Read the model definition and answer for the solid it produces. Units are mm, in the model's axes. Round coordinates to 2 decimals unless told otherwise and drop trailing zeros. One line per item, written item: value. Start each with the question number.
1. Consider line 1 (X direction, y = 77.5, z = 1.5); line 2 (Y direction, x = -30, z = 4.25); line 3 (Y direction, x = -64.5, z = 1.25). Determine where each line is inside the solid, lowest interval first.
2. The mould has two halves that part along Y. Classify faces 1 (the face through (-27, 109, 0.2)), 2 (the face through (-27, 100, 0.2)), 3 (the face through (3.05, -40.42, 4.45)), 4 (the face through (2.93, 118.42, 4.45)): released by +Y, released by -Y, zero draft, split by the parting line, or undercut.
3. Flat-ended cylindrical pins translate along their axes: pin 1 Ø3 at (y, z) = (-12, 5) entering from +X; pin 2 Ø1.1 at (x, z) = (-19.5, 4.5) entering from -Y; pin 3 Ø0.6 at (y, z) = (-42, 4.5) entering from -X. Find the tip coordinate at first contact, or state that the pin passes through.
from build123d import *

# Parameters (mm, degrees)
EXTRUDE_2_DEPTH     = 7.99
FILLET_4_R          = 1
EXTRUDE_4_DEPTH     = 0.7
SKETCH_13_R         = 0.94846709
CUT_EXTRUDE_2_DEPTH = 1
CUT_EXTRUDE_3_DEPTH = 1.5
CUT_EXTRUDE_4_DEPTH = 1.5
CUT_EXTRUDE_6_DEPTH = 0.2


with BuildPart() as part:
    # 草图1 → 凸台-拉伸2 (new body)
    with BuildSketch(Plane.XY):
        with BuildLine():
            Line((-62.348303156, 120.705678339), (-2.668303156, 120.705678339))
            ThreePointArc((-2.668303156, 120.705678339), (2.988551094, 118.362532589), (5.331696844, 112.705678339))
            Line((5.331696844, 112.705678339), (5.331696844, -34.824321661))
            ThreePointArc((5.331696844, -34.824321661), (2.988551094, -40.48117591), (-2.668303156, -42.824321661))
            Line((-2.668303156, -42.824321661), (-62.348303156, -42.824321661))
            ThreePointArc((-62.348303156, -42.824321661), (-68.005157405, -40.48117591), (-70.348303156, -34.824321661))
            Line((-70.348303156, -34.824321661), (-70.348303156, 112.705678339))
            ThreePointArc((-70.348303156, 112.705678339), (-68.005157405, 118.362532589), (-62.348303156, 120.705678339))
        make_face()
    extrude(amount=EXTRUDE_2_DEPTH)

    # 圆角4
    fillet_4_edges = [part.edges().sort_by_distance(p)[0] for p in [
        (5.331696844, 38.940678339, 0),
        (2.988551094, -40.48117591, 0),
        (-32.508303156, -42.824321661, 0),
        (-68.005157405, -40.48117591, 0),
        (-70.348303156, 38.940678339, 0),
        (-68.005157405, 118.362532589, 0),
        (-32.508303156, 120.705678339, 0),
        (2.988551094, 118.362532589, 0),
    ]]
    fillet(fillet_4_edges, radius=FILLET_4_R)

    # 草图7 → 凸台-拉伸4 (add)
    with BuildSketch(Plane(origin=(5.331696844, -15.049624304, 0), x_dir=(0, 0, -1), z_dir=(1, 0, 0))):
        with BuildLine():
            Line((-4.598017409, 67.245409355), (-4.480245782, 67.245409355))
            ThreePointArc((-4.480245782, 67.245409355), (-3.41958561, 66.806069527), (-2.980245782, 65.745409355))
            Line((-2.980245782, 65.745409355), (-2.980245782, 58.745409355))
            ThreePointArc((-2.980245782, 58.745409355), (-3.41958561, 57.684749184), (-4.480245782, 57.245409355))
            Line((-4.480245782, 57.245409355), (-4.598017409, 57.245409355))
            ThreePointArc((-4.598017409, 57.245409355), (-5.658677581, 57.684749184), (-6.098017409, 58.745409355))
            Line((-6.098017409, 58.745409355), (-6.098017409, 65.745409355))
            ThreePointArc((-6.098017409, 65.745409355), (-5.658677581, 66.806069527), (-4.598017409, 67.245409355))
        make_face()
        with BuildLine():
            Line((-4.653163904, 89.782491483), (-4.535392277, 89.782491483))
            ThreePointArc((-4.535392277, 89.782491483), (-3.474732105, 89.343151655), (-3.035392277, 88.282491483))
            Line((-3.035392277, 88.282491483), (-3.035392277, 74.219011632))
            ThreePointArc((-3.035392277, 74.219011632), (-3.474732105, 73.15835146), (-4.535392277, 72.719011632))
            Line((-4.535392277, 72.719011632), (-4.653163904, 72.719011632))
            ThreePointArc((-4.653163904, 72.719011632), (-5.713824076, 73.15835146), (-6.153163904, 74.219011632))
            Line((-6.153163904, 74.219011632), (-6.153163904, 88.282491483))
            ThreePointArc((-6.153163904, 88.282491483), (-5.713824076, 89.343151655), (-4.653163904, 89.782491483))
        make_face()
    extrude(amount=EXTRUDE_4_DEPTH)

    # 草图13 → 切除-拉伸2 (cut)
    with BuildSketch(Plane.XZ.offset(42.824321661)):
        with Locations(Location((-59.16469345, 4.443353111, 0), (0, 0, 270))):
            Circle(SKETCH_13_R)
    extrude(amount=-CUT_EXTRUDE_2_DEPTH, mode=Mode.SUBTRACT)

    # 草图14 → 切除-拉伸3 (cut)
    with BuildSketch(Plane.XZ.offset(42.824321661)):
        with BuildLine():
            Line((-35.262920742, 5.531025734), (-28.155701295, 5.531025734))
            ThreePointArc((-28.155701295, 5.531025734), (-27.660726548, 5.32600048), (-27.455701295, 4.831025734))
            Line((-27.455701295, 4.831025734), (-27.455701295, 3.72612223))
            ThreePointArc((-27.455701295, 3.72612223), (-27.660726548, 3.231147483), (-28.155701295, 3.02612223))
            Line((-28.155701295, 3.02612223), (-35.262920742, 3.02612223))
            ThreePointArc((-35.262920742, 3.02612223), (-35.757895489, 3.231147483), (-35.962920742, 3.72612223))
            Line((-35.962920742, 3.72612223), (-35.962920742, 4.831025734))
            ThreePointArc((-35.962920742, 4.831025734), (-35.757895489, 5.32600048), (-35.262920742, 5.531025734))
        make_face()
    extrude(amount=-CUT_EXTRUDE_3_DEPTH, mode=Mode.SUBTRACT)

    # 草图16 → 切除-拉伸4 (cut)
    with BuildSketch(Plane(origin=(0, -42.824321661, 0), x_dir=(-1, 0, 0), z_dir=(0, -1, 0))):
        with BuildLine():
            Line((16.936652763, -5.482735831), (16.77451846, -5.482735831))
            ThreePointArc((16.77451846, -5.482735831), (16.350254392, -5.3069999), (16.17451846, -4.882735831))
            Line((16.17451846, -4.882735831), (16.17451846, -3.642771963))
            ThreePointArc((16.17451846, -3.642771963), (16.350254392, -3.218507894), (16.77451846, -3.042771963))
            Line((16.77451846, -3.042771963), (16.936652763, -3.042771963))
            ThreePointArc((16.936652763, -3.042771963), (17.360916831, -3.218507894), (17.536652763, -3.642771963))
            Line((17.536652763, -3.642771963), (17.536652763, -4.882735831))
            ThreePointArc((17.536652763, -4.882735831), (17.360916831, -5.3069999), (16.936652763, -5.482735831))
        make_face()
        with BuildLine():
            Line((19.482830663, -5.466086098), (19.320696361, -5.466086098))
            ThreePointArc((19.320696361, -5.466086098), (18.896432292, -5.290350167), (18.720696361, -4.866086098))
            Line((18.720696361, -4.866086098), (18.720696361, -3.62612223))
            ThreePointArc((18.720696361, -3.62612223), (18.896432292, -3.201858161), (19.320696361, -3.02612223))
            Line((19.320696361, -3.02612223), (19.482830663, -3.02612223))
            ThreePointArc((19.482830663, -3.02612223), (19.907094732, -3.201858161), (20.082830663, -3.62612223))
            Line((20.082830663, -3.62612223), (20.082830663, -4.866086098))
            ThreePointArc((20.082830663, -4.866086098), (19.907094732, -5.290350167), (19.482830663, -5.466086098))
        make_face()
        with BuildLine():
            Line((14.704169667, -5.495191066), (14.542035364, -5.495191066))
            ThreePointArc((14.542035364, -5.495191066), (14.117771296, -5.319455135), (13.942035364, -4.895191066))
            Line((13.942035364, -4.895191066), (13.942035364, -3.655227198))
            ThreePointArc((13.942035364, -3.655227198), (14.117771296, -3.230963129), (14.542035364, -3.055227198))
            Line((14.542035364, -3.055227198), (14.704169667, -3.055227198))
            ThreePointArc((14.704169667, -3.055227198), (15.128433735, -3.230963129), (15.304169667, -3.655227198))
            Line((15.304169667, -3.655227198), (15.304169667, -4.895191066))
            ThreePointArc((15.304169667, -4.895191066), (15.128433735, -5.319455135), (14.704169667, -5.495191066))
        make_face()
        with BuildLine():
            Line((-17.076276663, -1.219981934), (-17.238410965, -1.219981934))
            ThreePointArc((-17.238410965, -1.219981934), (-17.662675034, -1.044246003), (-17.838410965, -0.619981934))
            Line((-17.838410965, -0.619981934), (-17.838410965, 0.619981934))
            ThreePointArc((-17.838410965, 0.619981934), (-17.662675034, 1.044246003), (-17.238410965, 1.219981934))
            Line((-17.238410965, 1.219981934), (-17.076276663, 1.219981934))
            ThreePointArc((-17.076276663, 1.219981934), (-16.652012594, 1.044246003), (-16.476276663, 0.619981934))
            Line((-16.476276663, 0.619981934), (-16.476276663, -0.619981934))
            ThreePointArc((-16.476276663, -0.619981934), (-16.652012594, -1.044246003), (-17.076276663, -1.219981934))
        make_face()
        with BuildLine():
            Line((12.291999198, -5.500173127), (12.129864896, -5.500173127))
            ThreePointArc((12.129864896, -5.500173127), (11.705600827, -5.324437196), (11.529864896, -4.900173127))
            Line((11.529864896, -4.900173127), (11.529864896, -3.660209259))
            ThreePointArc((11.529864896, -3.660209259), (11.705600827, -3.23594519), (12.129864896, -3.060209259))
            Line((12.129864896, -3.060209259), (12.291999198, -3.060209259))
            ThreePointArc((12.291999198, -3.060209259), (12.716263267, -3.23594519), (12.891999198, -3.660209259))
            Line((12.891999198, -3.660209259), (12.891999198, -4.900173127))
            ThreePointArc((12.891999198, -4.900173127), (12.716263267, -5.324437196), (12.291999198, -5.500173127))
        make_face()
        with BuildLine():
            Line((9.984598284, -5.482371765), (9.822463982, -5.482371765))
            ThreePointArc((9.822463982, -5.482371765), (9.398199913, -5.306635834), (9.222463982, -4.882371765))
            Line((9.222463982, -4.882371765), (9.222463982, -3.642407897))
            ThreePointArc((9.222463982, -3.642407897), (9.398199913, -3.218143828), (9.822463982, -3.042407897))
            Line((9.822463982, -3.042407897), (9.984598284, -3.042407897))
            ThreePointArc((9.984598284, -3.042407897), (10.408862353, -3.218143828), (10.584598284, -3.642407897))
            Line((10.584598284, -3.642407897), (10.584598284, -4.882371765))
            ThreePointArc((10.584598284, -4.882371765), (10.408862353, -5.306635834), (9.984598284, -5.482371765))
        make_face()
        with BuildLine():
            Line((7.784966211, -5.482371765), (7.622831908, -5.482371765))
            ThreePointArc((7.622831908, -5.482371765), (7.19856784, -5.306635834), (7.022831908, -4.882371765))
            Line((7.022831908, -4.882371765), (7.022831908, -3.642407897))
            ThreePointArc((7.022831908, -3.642407897), (7.19856784, -3.218143828), (7.622831908, -3.042407897))
            Line((7.622831908, -3.042407897), (7.784966211, -3.042407897))
            ThreePointArc((7.784966211, -3.042407897), (8.209230279, -3.218143828), (8.384966211, -3.642407897))
            Line((8.384966211, -3.642407897), (8.384966211, -4.882371765))
            ThreePointArc((8.384966211, -4.882371765), (8.209230279, -5.306635834), (7.784966211, -5.482371765))
        make_face()
        with BuildLine():
            Line((40.445771945, -5.535278568), (40.283637643, -5.535278568))
            ThreePointArc((40.283637643, -5.535278568), (39.859373574, -5.359542637), (39.683637643, -4.935278568))
            Line((39.683637643, -4.935278568), (39.683637643, -3.6953147))
            ThreePointArc((39.683637643, -3.6953147), (39.859373574, -3.271050631), (40.283637643, -3.0953147))
            Line((40.283637643, -3.0953147), (40.445771945, -3.0953147))
            ThreePointArc((40.445771945, -3.0953147), (40.870036014, -3.271050631), (41.045771945, -3.6953147))
            Line((41.045771945, -3.6953147), (41.045771945, -4.935278568))
            ThreePointArc((41.045771945, -4.935278568), (40.870036014, -5.359542637), (40.445771945, -5.535278568))
        make_face()
    extrude(amount=-CUT_EXTRUDE_4_DEPTH, mode=Mode.SUBTRACT)

    # 草图18 → 切除-拉伸6 (cut)
    with BuildSketch(Plane(origin=(0, 0, 0), x_dir=(-1, 0, 0), z_dir=(0, 0, -1))):
        with BuildLine():
            Line((25.012472849, 102.092998362), (29.012472849, 102.092998362))
            ThreePointArc((29.012472849, 102.092998362), (29.36602624, 101.946551752), (29.512472849, 101.592998362))
            Line((29.512472849, 101.592998362), (29.512472849, 97.592998362))
            ThreePointArc((29.512472849, 97.592998362), (29.36602624, 97.239444971), (29.012472849, 97.092998362))
            Line((29.012472849, 97.092998362), (25.012472849, 97.092998362))
            ThreePointArc((25.012472849, 97.092998362), (24.658919458, 97.239444971), (24.512472849, 97.592998362))
            Line((24.512472849, 97.592998362), (24.512472849, 101.592998362))
            ThreePointArc((24.512472849, 101.592998362), (24.658919458, 101.946551752), (25.012472849, 102.092998362))
        make_face()
        with BuildLine():
            Line((24.948975022, 111.702722859), (28.948975022, 111.702722859))
            ThreePointArc((28.948975022, 111.702722859), (29.302528413, 111.55627625), (29.448975022, 111.202722859))
            Line((29.448975022, 111.202722859), (29.448975022, 107.202722859))
            ThreePointArc((29.448975022, 107.202722859), (29.302528413, 106.849169469), (28.948975022, 106.702722859))
            Line((28.948975022, 106.702722859), (24.948975022, 106.702722859))
            ThreePointArc((24.948975022, 106.702722859), (24.595421632, 106.849169469), (24.448975022, 107.202722859))
            Line((24.448975022, 107.202722859), (24.448975022, 111.202722859))
            ThreePointArc((24.448975022, 111.202722859), (24.595421632, 111.55627625), (24.948975022, 111.702722859))
        make_face()
    extrude(amount=-CUT_EXTRUDE_6_DEPTH, mode=Mode.SUBTRACT)


solid = part.part
Answer:
1. line 1: -70.35 to 5.33
1. line 2: -41.32 to 120.71
1. line 3: -42.53 to 120.41
2. face 1: undercut
2. face 2: undercut
2. face 3: released by -Y
2. face 4: released by +Y
3. pin 1: x = 5.33
3. pin 2: y = -41.32
3. pin 3: x = -66.44
